Geometry: final body of the model. Coordinates: model frame, mm. A direction names the side the tool comes from. Round coordinates to 2 decimals unless told otherwise and drop trailing zeros. Write each loop counter-clockwise with the first axis right and the second up, starting at its lowest first coordinate (ties: lowest second). Pieces come first, ordered by that corner, then holes. Notation, with made-up numbers: M -9,41 L 50,41 A4 ccw 50,48 Z; hole C 60.25,-35.75 d10. An arc over 180 degrees is marked long. Use one line per item in the form item = value. Start each with the question number.
Item 1: Reachability of faces 5 (the flat face through (25, 25, 18)), 6 (the flat face through (22, 23, 17)), 7 (the flat face through (5.835, 11.042, 8.036)) from +Z, -Z, +X, -X, +Y, -Y: full face, straight path, thin tool, end or side. Return the list, or none.
Item 2: Section query B-B (y = 5). State how many separate pieces and enclosed holes the cut face has, and give its area (3 significant figures).
Item 3: Section query A-A (z = 1.5). Return loops of the section in (x, y), and give its area (3 significant figures).
Item 4: Pin query (flat end, axial travel): pin 1 Ø3 at (y, z) = (25, 11) entering from +X; pin 2 Ø6.5 at (x, z) = (23.5, 12.5) entering from +Y; pin 3 Ø9 at (x, y) = (22.5, 24.5) entering from -Z. Return the tip coordinate at first contact, or that it passes through.
Item 5: Ray query, probe 1 along Y at (x, z) = (20, 1.75); probe 2 along Z at (x, y) = (28.5, 19.5); probe 3 along Y at (x, z) = (13, 17.75). Return the intervals inside material, ascending.
Item 6: Pull-direction query (Z, two-part tool) for faces 1 (the flat face through (0, 15, 10)), 2 (the cylindrical face through (22.353, 11.851, 14.324)), 3 (the flat face through (14.96, 5.88, 7.96)), 4 (the flat face through (15, 12, 0)); classes: pulls with the +Z half, pulls with the -Z half, needs draft (parallel to the pull), parting line crosses it, or undercut.
from build123d import *

# Parameters (mm, degrees)
CYLINDER001_R        = 3
CYLINDER001_DEPTH    = 40
CYLINDER_R           = 1.7
CYLINDER_DEPTH       = 40
FUSION001_ROLL_ANGLE = -60
FUSION_PITCH_ANGLE   = 60
BOX001_W             = 18
BOX001_H             = 19
BOX001_DEPTH         = 20
BOX_W                = 30
BOX_H                = 30
BOX_DEPTH            = 20
CHAMFER_SIZE         = 10


with BuildPart() as cylinder001:
    # Cylinder001 → Cylinder001 (new body)
    with BuildSketch(Plane.XY.offset(16)):
        Circle(CYLINDER001_R)
    extrude(amount=CYLINDER001_DEPTH)


with BuildPart() as cylinder:
    # Cylinder → Cylinder (new body)
    with BuildSketch(Plane.XY):
        Circle(CYLINDER_R)
    extrude(amount=CYLINDER_DEPTH)


with BuildPart() as screw001:
    # Fusion001 base: copy of Cylinder
    add(cylinder.part)

    # Fusion001: union Cylinder001
    add(cylinder001.part)


with BuildPart() as screw001_1:
    # Fusion001 roll: moved
    add(screw001.part.rotate(Axis((0, 0, 0), (1, 0, 0)), FUSION001_ROLL_ANGLE))


with BuildPart() as screw001_2:
    # Fusion001 placement: moved
    add(screw001_1.part.moved(Location((13, -8, 0))))


with BuildPart() as fusion002:
    # Fusion base: copy of Cylinder
    add(cylinder.part)

    # Fusion: union Cylinder001
    add(cylinder001.part)


with BuildPart() as fusion002_1:
    # Fusion pitch: moved
    add(fusion002.part.rotate(Axis((0, 0, 0), (0, 1, 0)), FUSION_PITCH_ANGLE))


with BuildPart() as fusion002_2:
    # Fusion placement: moved
    add(fusion002_1.part.moved(Location((-8, 13, 0))))

    # Fusion002: union screw001
    add(screw001_2.part)


with BuildPart() as cube001:
    # Box001 → Box001 (new body)
    with BuildSketch(Plane(origin=(17, 19, -3), x_dir=(1, 0, 0), z_dir=(0, 0, 1))):
        with Locations((9, 9.5)):
            Rectangle(BOX001_W, BOX001_H)
    extrude(amount=BOX001_DEPTH)


with BuildPart() as cut001:
    # Box → Box (new body)
    with BuildSketch(Plane.XY):
        with Locations((15, 15)):
            Rectangle(BOX_W, BOX_H)
    extrude(amount=BOX_DEPTH)

    # Chamfer
    chamfer_edges = [cut001.edges().sort_by_distance(p)[0] for p in [
        (30, 30, 10),
    ]]
    chamfer(chamfer_edges, length=CHAMFER_SIZE)

    # Cut: cut Cube001
    add(cube001.part, mode=Mode.SUBTRACT)

    # Cut001: cut Fusion002
    add(fusion002_2.part, mode=Mode.SUBTRACT)


solid = cut001.part
Working result:
q1.face_5 = +Z, -Z, +X, +Y
q1.face_6 = -Z, +X, +Y
q1.face_7 = none
q2.separate_pieces = 1
q2.enclosed_holes = 2
q2.area = 584 mm²
q3.outline = M 0,0 L 30,0 L 30,19 L 17,19 L 17,30 L 0,30 Z
q3.area = 757 mm²
q4.pin_1 = 17
q4.pin_2 = 19
q4.pin_3 = 17
q5.probe_1 = 0 to 19
q5.probe_2 = 17 to 20
q5.probe_3 = 0 to 16.74, 28.74 to 30
q6.face_1 = needs draft
q6.face_2 = undercut
q6.face_3 = undercut
q6.face_4 = pulls with the -Z half
